Can you work these out from the model? Positions are in its coordinate system, mm. Give positions to 0.01 mm unless a question says otherwise; leave off trailing zeros. Loops run counter-clockwise (first coordinate to the right, second up) from the corner with the lowest first, then second, coordinate; pieces in that order, holes last. Notation, with made-up numbers: (87.5, 21.5) -> (118.5, 21.5) arc R19 ccw to (118.5, 30.5) -> close; hole circle Ø4 at (39.5, 29). An arc over 180 degrees is marked (long way). One line per question, with ' | ' between items.
from build123d import *

# Parameters (mm, degrees)
CROQUIS3_R              = 85
SALIENTE_EXTRUIR1_DEPTH = 4
CORTAR_EXTRUIR1_START   = -4
CORTAR_EXTRUIR1_DEPTH   = 4
CROQUIS5_R              = 15
CORTAR_EXTRUIR2_DEPTH   = 4
CROQUIS6_R              = 15
CORTAR_EXTRUIR3_DEPTH   = 4


with BuildPart() as part:
    # Croquis3 → Saliente-Extruir1 (new body)
    with BuildSketch(Plane.XY):
        Circle(CROQUIS3_R)
    extrude(amount=SALIENTE_EXTRUIR1_DEPTH)

    # Croquis4 → Cortar-Extruir1 (cut)
    with BuildSketch(Plane.XY.offset(4).offset(CORTAR_EXTRUIR1_START)):
        with BuildLine():
            ThreePointArc((51.744720944, 67.435034325), (32.528091082, 78.52976054), (11.094725556, 84.27281332))
            ThreePointArc((11.094725556, 84.27281332), (16.790892389, 81.996657131), (20.705523608, 77.274066103))
            ThreePointArc((20.705523608, 77.274066103), (28.813811378, 69.562694213), (40, 69.282032303))
            ThreePointArc((40, 69.282032303), (46.107437706, 69.853346275), (51.744720944, 67.435034325))
        make_face()
        with BuildLine():
            ThreePointArc((-20.705523608, 77.274066103), (-10.442095378, 79.31558891), (0, 80))
            ThreePointArc((0, 80), (5.003539158, 83.548491243), (11.094725556, 84.27281332))
            ThreePointArc((11.094725556, 84.27281332), (-11.094726837, 84.272813151), (-32.52809195, 78.529760181))
            ThreePointArc((-32.52809195, 78.529760181), (-26.456988918, 79.406634265), (-20.705523608, 77.274066103))
        make_face()
        with BuildLine():
            ThreePointArc((-20.705523608, 77.274066103), (-9.827854473, 74.649966033), (0, 80))
            ThreePointArc((0, 80), (-10.442095378, 79.31558891), (-20.705523608, 77.274066103))
        make_face()
        with BuildLine():
            ThreePointArc((-40, 69.282032303), (-37.441053421, 74.856885666), (-32.52809195, 78.529760181))
            ThreePointArc((-32.52809195, 78.529760181), (-51.744721795, 67.435033672), (-67.435034299, 51.744720978))
            ThreePointArc((-67.435034299, 51.744720978), (-62.615741826, 55.539667962), (-56.568542495, 56.568542495))
            ThreePointArc((-56.568542495, 56.568542495), (-48.700914321, 63.468267223), (-40, 69.282032303))
        make_face()
        with BuildLine():
            ThreePointArc((-56.568542495, 56.568542495), (-45.836154655, 59.73483974), (-40, 69.282032303))
            ThreePointArc((-40, 69.282032303), (-48.700914321, 63.468267223), (-56.568542495, 56.568542495))
        make_face()
        with BuildLine():
            ThreePointArc((-69.282032303, 40), (-69.853346272, 46.107437728), (-67.435034299, 51.744720978))
            ThreePointArc((-67.435034299, 51.744720978), (-78.529760525, 32.528091121), (-84.272813315, 11.094725594))
            ThreePointArc((-84.272813315, 11.094725594), (-81.996657119, 16.790892405), (-77.274066103, 20.705523608))
            ThreePointArc((-77.274066103, 20.705523608), (-73.910362601, 30.614674589), (-69.282032303, 40))
        make_face()
        with BuildLine():
            ThreePointArc((-77.274066103, 20.705523608), (-69.562694213, 28.813811378), (-69.282032303, 40))
            ThreePointArc((-69.282032303, 40), (-73.910362601, 30.614674589), (-77.274066103, 20.705523608))
        make_face()
        with BuildLine():
            ThreePointArc((-80, 0), (-83.54849125, 5.003539176), (-84.272813315, 11.094725594))
            ThreePointArc((-84.272813315, 11.094725594), (-84.272813233, -11.094726218), (-78.529760644, -32.528090833))
            ThreePointArc((-78.529760644, -32.528090833), (-79.406634201, -26.456988317), (-77.274066103, -20.705523608))
            ThreePointArc((-77.274066103, -20.705523608), (-79.31558891, -10.442095378), (-80, 0))
        make_face()
        with BuildLine():
            ThreePointArc((-77.274066103, -20.705523608), (-74.649966033, -9.827854473), (-80, 0))
            ThreePointArc((-80, 0), (-79.31558891, -10.442095378), (-77.274066103, -20.705523608))
        make_face()
        with BuildLine():
            ThreePointArc((-69.282032303, -40), (-74.856886137, -37.441053042), (-78.529760644, -32.528090833))
            ThreePointArc((-78.529760644, -32.528090833), (-67.435033831, -51.744721588), (-51.744720432, -67.435034718))
            ThreePointArc((-51.744720432, -67.435034718), (-55.539667823, -62.61574214), (-56.568542495, -56.568542495))
            ThreePointArc((-56.568542495, -56.568542495), (-63.468267223, -48.700914321), (-69.282032303, -40))
        make_face()
        with BuildLine():
            ThreePointArc((-56.568542495, -56.568542495), (-59.73483974, -45.836154655), (-69.282032303, -40))
            ThreePointArc((-69.282032303, -40), (-63.468267223, -48.700914321), (-56.568542495, -56.568542495))
        make_face()
        with BuildLine():
            ThreePointArc((-40, -69.282032303), (-46.107437388, -69.853346325), (-51.744720432, -67.435034718))
            ThreePointArc((-51.744720432, -67.435034718), (-32.528090639, -78.529760724), (-11.094725244, -84.272813361))
            ThreePointArc((-11.094725244, -84.272813361), (-16.790892262, -81.996657223), (-20.705523608, -77.274066103))
            ThreePointArc((-20.705523608, -77.274066103), (-30.614674589, -73.910362601), (-40, -69.282032303))
        make_face()
        with BuildLine():
            ThreePointArc((-20.705523608, -77.274066103), (-28.813811378, -69.562694213), (-40, -69.282032303))
            ThreePointArc((-40, -69.282032303), (-30.614674589, -73.910362601), (-20.705523608, -77.274066103))
        make_face()
        with BuildLine():
            ThreePointArc((-11.094725244, -84.272813361), (11.09472631, -84.272813221), (32.528090677, -78.529760708))
            ThreePointArc((32.528090677, -78.529760708), (26.456988234, -79.406634192), (20.705523608, -77.274066103))
            ThreePointArc((20.705523608, -77.274066103), (10.442095378, -79.31558891), (0, -80))
            ThreePointArc((0, -80), (-5.003539011, -83.548491186), (-11.094725244, -84.272813361))
        make_face()
        with BuildLine():
            ThreePointArc((0, -80), (10.442095378, -79.31558891), (20.705523608, -77.274066103))
            ThreePointArc((20.705523608, -77.274066103), (9.827854473, -74.649966033), (0, -80))
        make_face()
        with BuildLine():
            ThreePointArc((40, -69.282032303), (48.700914321, -63.468267223), (56.568542495, -56.568542495))
            ThreePointArc((56.568542495, -56.568542495), (45.836154655, -59.73483974), (40, -69.282032303))
        make_face()
        with BuildLine():
            ThreePointArc((32.528090677, -78.529760708), (51.74472148, -67.435033914), (67.435034654, -51.744720516))
            ThreePointArc((67.435034654, -51.744720516), (62.615742092, -55.539667844), (56.568542495, -56.568542495))
            ThreePointArc((56.568542495, -56.568542495), (48.700914321, -63.468267223), (40, -69.282032303))
            ThreePointArc((40, -69.282032303), (37.441052989, -74.856886202), (32.528090677, -78.529760708))
        make_face()
        with BuildLine():
            ThreePointArc((67.435034654, -51.744720516), (78.529760638, -32.528090847), (84.272813316, -11.094725585))
            ThreePointArc((84.272813316, -11.094725585), (81.996657122, -16.790892401), (77.274066103, -20.705523608))
            ThreePointArc((77.274066103, -20.705523608), (73.910362601, -30.614674589), (69.282032303, -40))
            ThreePointArc((69.282032303, -40), (69.853346317, -46.10743744), (67.435034654, -51.744720516))
        make_face()
        with BuildLine():
            ThreePointArc((69.282032303, -40), (73.910362601, -30.614674589), (77.274066103, -20.705523608))
            ThreePointArc((77.274066103, -20.705523608), (69.562694213, -28.813811378), (69.282032303, -40))
        make_face()
        with BuildLine():
            ThreePointArc((85, 0), (83.36674891, 16.582676993), (78.529760559, 32.528091037))
            ThreePointArc((78.529760559, 32.528091037), (79.406634213, 26.456988427), (77.274066103, 20.705523608))
            ThreePointArc((77.274066103, 20.705523608), (79.31558891, 10.442095378), (80, 0))
            ThreePointArc((80, 0), (83.548491248, -5.003539172), (84.272813316, -11.094725585))
            ThreePointArc((84.272813316, -11.094725585), (84.8180085, -5.559265605), (85, 0))
        make_face()
        with BuildLine():
            ThreePointArc((80, 0), (79.31558891, 10.442095378), (77.274066103, 20.705523608))
            ThreePointArc((77.274066103, 20.705523608), (74.649966033, 9.827854473), (80, 0))
        make_face()
        with BuildLine():
            ThreePointArc((78.529760559, 32.528091037), (67.43503396, 51.74472142), (51.744720944, 67.435034325))
            ThreePointArc((51.744720944, 67.435034325), (55.539667954, 62.615741846), (56.568542495, 56.568542495))
            ThreePointArc((56.568542495, 56.568542495), (63.468267223, 48.700914321), (69.282032303, 40))
            ThreePointArc((69.282032303, 40), (74.856886051, 37.441053111), (78.529760559, 32.528091037))
        make_face()
        with BuildLine():
            ThreePointArc((69.282032303, 40), (63.468267223, 48.700914321), (56.568542495, 56.568542495))
            ThreePointArc((56.568542495, 56.568542495), (59.73483974, 45.836154655), (69.282032303, 40))
        make_face()
    extrude(amount=CORTAR_EXTRUIR1_DEPTH, mode=Mode.SUBTRACT)

    # Croquis5 → Cortar-Extruir2 (cut)
    with BuildSketch(Plane.XY.offset(4)):
        Circle(CROQUIS5_R)
    extrude(amount=-CORTAR_EXTRUIR2_DEPTH, mode=Mode.SUBTRACT)

    # Croquis6 → Cortar-Extruir3 (cut)
    with BuildSketch(Plane.XY.offset(4)):
        with Locations((14.406905689, 34.781347106)):
            Circle(CROQUIS6_R)
        with Locations((34.781347106, -14.406905689)):
            Circle(CROQUIS6_R)
        with Locations((-14.406905689, -34.781347106)):
            Circle(CROQUIS6_R)
        with Locations((-34.781347106, 14.406905689)):
            Circle(CROQUIS6_R)
    extrude(amount=-CORTAR_EXTRUIR3_DEPTH, mode=Mode.SUBTRACT)


solid = part.part
Q1. If I drill on probe 1 along Y at (x, z) = (-11, 0.9); probe 2 along Y at (x, z) = (-5, 1.5); probe 3 along X at (y, z) = (-3, 3.4), over which ranges is the centre line in solid material (lowest first)? Write a range as from..to.
Entries:
probe 1: -84.28..-49.39, -20.17..-10.2, 10.2..74.54 | probe 2: -83.55..-46.47, -23.1..-14.14, 14.14..76.11 | probe 3: -77.28..-14.7, 14.7..25.04, 44.52..82.56
Q2. For pin 1 Ø1 at (x, z) = (-38, 2) entering from +Y; pin 2 Ø1 at (x, z) = (5, 0.5) entering from -Y; pin 3 Ø1.5 at (y, z) = (-59.5, 1.5) entering from +X, each with a flat end and sliding along its axis, tell me the tip position at first contact or that it passes through.
Entries:
pin 1: y = 74.78 | pin 2: y = -76.37 | pin 3: x = 47.28
Q3. If we mould it in two halves opening along X, with no side actions, what happens to faces 1 (the face through (-74.63, -9.99, 1.97)), 2 (the face through (9.99, -74.63, 1.97)), 3 (the face through (18, 1, 4))? For each: pulls with the +X half, pulls with the -X half, needs draft (parallel to the pull), parting line crosses it, or undercut.
Entries:
face 1: pulls with the -X half | face 2: undercut | face 3: needs draft
Q4. If we section it at A-A (x = 46.5): Write out the boundary of the cut face in (y, z), plus the area to 3 significant figures.
Entries:
outline: (-59.25, 0) -> (-23.77, 0) -> (-23.77, 4) -> (-59.25, 4) -> close; (-5.04, 0) -> (69.79, 0) -> (69.79, 4) -> (-5.04, 4) -> close | area: 441 mm²
Q5. If we section it at B-B (x = -25): Write out the boundary of the cut face in (y, z), plus the area to 3 significant figures.
Entries:
outline: (-71.83, 0) -> (-45.4, 0) -> (-45.4, 4) -> (-71.83, 4) -> close; (-24.16, 0) -> (3.03, 0) -> (3.03, 4) -> (-24.16, 4) -> close; (25.78, 0) -> (79.16, 0) -> (79.16, 4) -> (25.78, 4) -> close | area: 428 mm²
Q6. If we section it at D-D (x = -42): Write out the boundary of the cut face in (y, z).
Entries:
outline: (-69.81, 0) -> (1.26, 0) -> (1.26, 4) -> (-69.81, 4) -> close; (27.56, 0) -> (64.02, 0) -> (64.02, 4) -> (27.56, 4) -> close
Q7. If we section it at C-C (z = 1): State how many separate pieces and enclosed holes the cut face has, plus the area to 3 significant figures.
Entries:
separate pieces: 1 | enclosed holes: 5 | area: 16,700 mm²
